```python
from build123d import *

# Parameters (mm, degrees)
F0_W     = 40
F0_H     = 6
F1_DEPTH = 3
F3_DEPTH = 45
F4_W     = 40
F4_H     = 6
F5_DEPTH = 3
F6_R     = 1.55
F7_DEPTH = 51.001


with BuildPart() as f1:
    # F0 (on Front) → F1 (new body)
    with BuildSketch(Plane.XZ):
        Rectangle(F0_W, F0_H)
    extrude(amount=F1_DEPTH)

    # F2 (on face) → F3 (join)
    with BuildSketch(Plane.XZ.offset(3)):
        Polygon((1, -3), (3.527162, -1), (3.527162, 1), (1, 3), (-1, 3), (-3.527162, 1), (-3.527162, -1), (-1, -3), align=None)
    extrude(amount=F3_DEPTH)

    # F4 (on face) → F5 (join)
    with BuildSketch(Plane.XZ.offset(48)):
        Rectangle(F4_W, F4_H)
    extrude(amount=F5_DEPTH)

    # F6 (on face) → F7 (cut, through all)
    with BuildSketch(Plane(origin=(0, 0, 0), x_dir=(-1, 0, 0), z_dir=(0, 1, 0))):
        with Locations((-16, 0)):
            Circle(F6_R)
        with Locations((16, 0)):
            Circle(F6_R)
    extrude(amount=-F7_DEPTH, mode=Mode.SUBTRACT)


solid = f1.part
```
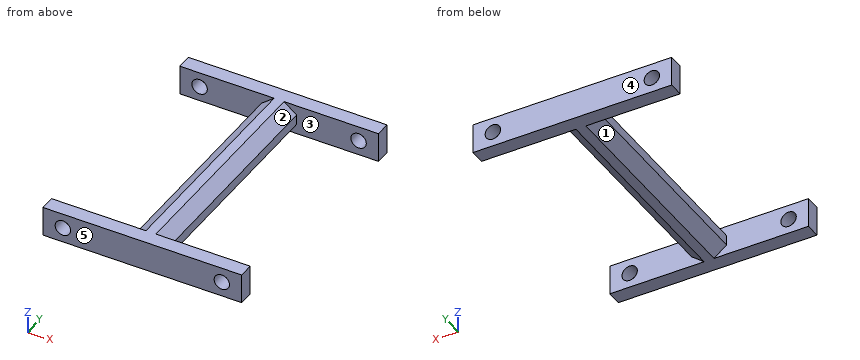
Design review of the part built by this model. Coordinates are the model's own, in mm. Face numbers are marked on the shaded views. A direction names the side the tool comes from. Give positions to 0.01 mm unless a question says otherwise; leave off trailing zeros. Write each loop counter-clockwise with the first axis right and the second up, starting at its lowest first coordinate (ties: lowest second). Pieces come first, ordered by that corner, then holes. Notation, with made-up numbers: (78.25, 31) - (90.25, 31) arc R33 ccw to (90.25, 62) - close; hole circle Ø9 at (-36, 53). An arc over 180 degrees is marked (long way). Return JSON: item names as keys, results as strings. Group by question number.
(1) Machinability: for the marked faces 1 and 2, which of the approach directions +Z, -Z, +X, -X, +Y, -Y give a long, thin tool a straight path to every point of the face, cutting with its end or side? Answer none if there is none.
(2) Insertion check: pin 1 (0.6 mm diameter, centred on y = -36, z = 0.5, fed in from +X); pin 2 (2 mm diameter, centred on y = -24, z = 0, fed in from -X). Each pin has a flat end and moves straight along its axis. Give the tip position at first contact, or say it passes through.
(3) We need section D-D, the plane x = -16. Give the boundary of the cut face in (y, z).
(4) We need section C-C, the plane y = -43. Give the boundary of the cut face in (x, z), then the cut area to 3 significant figures.
(5) We need section A-A, the plane x = -9. Give the boundary of the cut face in (y, z).
(6) Mouldability with a two-part tool opening along Y and no side actions: class the marked faces 3, 4 and 5 as +Y half, -Y half, draft (parallel to the pull), parting line (faces both ways), or undercut.
(7) We need section B-B, the plane z = 0. Give the boundary of the cut face in (x, y), then the cut area to 3 significant figures.
(8) To check wall thickness, follow probe 1 along Y at (x, z) = (9.5, -0.15); probe 2 along Z at (x, y) = (16, -49.3); probe 3 along X at (y, z) = (-8.5, -0.2). State the ranges of each line that lie inside material, in increasing order.
Reported:
{
 "1": {"face 1": "-Z, -X", "face 2": "+Z, +X"},
 "2": {"pin 1": "stops at x = 3.53", "pin 2": "stops at x = -3.53"},
 "3": {"outline": "(-51, -3) - (-48, -3) - (-48, -1.55) - (-51, -1.55) - close; (-51, 1.55) - (-48, 1.55) - (-48, 3) - (-51, 3) - close; (-3, -3) - (0, -3) - (0, -1.55) - (-3, -1.55) - close; (-3, 1.55) - (0, 1.55) - (0, 3) - (-3, 3) - close"},
 "4": {"outline": "(-3.53, -1) - (-1, -3) - (1, -3) - (3.53, -1) - (3.53, 1) - (1, 3) - (-1, 3) - (-3.53, 1) - close", "area": "32.2 mm2"},
 "5": {"outline": "(-51, -3) - (-48, -3) - (-48, 3) - (-51, 3) - close; (-3, -3) - (0, -3) - (0, 3) - (-3, 3) - close"},
 "6": {"face 3": "undercut", "face 4": "+Y half", "face 5": "-Y half"},
 "7": {"outline": "(-20, -51) - (-17.55, -51) - (-17.55, -48) - (-20, -48) - close; (-20, -3) - (-17.55, -3) - (-17.55, 0) - (-20, 0) - close; (-14.45, -51) - (14.45, -51) - (14.45, -48) - (3.53, -48) - (3.53, -3) - (14.45, -3) - (14.45, 0) - (-14.45, 0) - (-14.45, -3) - (-3.53, -3) - (-3.53, -48) - (-14.45, -48) - close; (17.55, -51) - (20, -51) - (20, -48) - (17.55, -48) - close; (17.55, -3) - (20, -3) - (20, 0) - (17.55, 0) - close", "area": "520 mm2"},
 "8": {"probe 1": "y = -51 to -48, -3 to 0", "probe 2": "z = -3 to -1.55, 1.55 to 3", "probe 3": "x = -3.53 to 3.53"}
}
